from build123d import *

# Parameters (mm, degrees)
SKETCH1_W                 = 100
SKETCH1_H                 = 75
BOSS_EXTRUDE1_DEPTH       = 3.5
F_6_0MM_DOWEL_HOLE5_D     = 6
F_6_0MM_DOWEL_HOLE5_DEPTH = 5.2
F_6_0MM_DOWEL_HOLE5_TIP   = 1.802581857
F_6_0MM_DOWEL_HOLE6_D     = 6
F_6_0MM_DOWEL_HOLE6_DEPTH = 5.2
F_6_0MM_DOWEL_HOLE6_TIP   = 1.802581857
F_6_0MM_DOWEL_HOLE7_D     = 6
F_6_0MM_DOWEL_HOLE7_DEPTH = 5.2
F_6_0MM_DOWEL_HOLE7_TIP   = 1.802581857
F_6_0MM_DOWEL_HOLE8_D     = 6
F_6_0MM_DOWEL_HOLE8_DEPTH = 5.2
F_6_0MM_DOWEL_HOLE8_TIP   = 1.802581857
F_6_0MM_DOWEL_HOLE9_D     = 6
F_6_0MM_DOWEL_HOLE10_D    = 6


with BuildPart() as part:
    # Sketch1 → Boss-Extrude1 (new body)
    with BuildSketch(Plane(origin=(0, 0, 0), x_dir=(1, 0, 0), z_dir=(0, 1, 0))):
        with Locations((-13.448964329, -14.251552142)):
            Rectangle(SKETCH1_W, SKETCH1_H)
    extrude(amount=BOSS_EXTRUDE1_DEPTH)

    # Ø6.0mm Dowel Hole5
    with Locations(Plane(origin=(-137.528418299, 0, 99.034606683), x_dir=(-1, 0, 0), z_dir=(0, -1, 0))):
        with Locations((-154.698850598, 100.900481409)):
            Hole(F_6_0MM_DOWEL_HOLE5_D / 2, depth=F_6_0MM_DOWEL_HOLE5_DEPTH)
            with Locations((0, 0, -(F_6_0MM_DOWEL_HOLE5_DEPTH + F_6_0MM_DOWEL_HOLE5_TIP / 2))):  # 118° drill point
                Cone(0, F_6_0MM_DOWEL_HOLE5_D / 2, F_6_0MM_DOWEL_HOLE5_TIP, mode=Mode.SUBTRACT)

    # Ø6.0mm Dowel Hole6
    with Locations(Plane(origin=(-137.528418299, 0, 99.034606683), x_dir=(-1, 0, 0), z_dir=(0, -1, 0))):
        with Locations((-121.736726509, 100.900481409)):
            Hole(F_6_0MM_DOWEL_HOLE6_D / 2, depth=F_6_0MM_DOWEL_HOLE6_DEPTH)
            with Locations((0, 0, -(F_6_0MM_DOWEL_HOLE6_DEPTH + F_6_0MM_DOWEL_HOLE6_TIP / 2))):  # 118° drill point
                Cone(0, F_6_0MM_DOWEL_HOLE6_D / 2, F_6_0MM_DOWEL_HOLE6_TIP, mode=Mode.SUBTRACT)

    # Ø6.0mm Dowel Hole7
    with Locations(Plane(origin=(-137.528418299, 0, 99.034606683), x_dir=(-1, 0, 0), z_dir=(0, -1, 0))):
        with Locations((-154.698850598, 68.255290468)):
            Hole(F_6_0MM_DOWEL_HOLE7_D / 2, depth=F_6_0MM_DOWEL_HOLE7_DEPTH)
            with Locations((0, 0, -(F_6_0MM_DOWEL_HOLE7_DEPTH + F_6_0MM_DOWEL_HOLE7_TIP / 2))):  # 118° drill point
                Cone(0, F_6_0MM_DOWEL_HOLE7_D / 2, F_6_0MM_DOWEL_HOLE7_TIP, mode=Mode.SUBTRACT)

    # Ø6.0mm Dowel Hole8
    with Locations(Plane(origin=(-137.528418299, 0, 99.034606683), x_dir=(-1, 0, 0), z_dir=(0, -1, 0))):
        with Locations((-121.736726509, 68.255290468)):
            Hole(F_6_0MM_DOWEL_HOLE8_D / 2, depth=F_6_0MM_DOWEL_HOLE8_DEPTH)
            with Locations((0, 0, -(F_6_0MM_DOWEL_HOLE8_DEPTH + F_6_0MM_DOWEL_HOLE8_TIP / 2))):  # 118° drill point
                Cone(0, F_6_0MM_DOWEL_HOLE8_D / 2, F_6_0MM_DOWEL_HOLE8_TIP, mode=Mode.SUBTRACT)

    # Ø6.0mm Dowel Hole9 (through all)
    with Locations(Plane(origin=(-137.528418299, 0, 99.034606683), x_dir=(-1, 0, 0), z_dir=(0, -1, 0))):
        with Locations((-93.346603373, 84.436908191)):
            Hole(F_6_0MM_DOWEL_HOLE9_D / 2)

    # Ø6.0mm Dowel Hole10 (through all)
    with Locations(Plane(origin=(-137.528418299, 0, 99.034606683), x_dir=(-1, 0, 0), z_dir=(0, -1, 0))):
        with Locations((-126.399729662, 84.576636181)):
            Hole(F_6_0MM_DOWEL_HOLE10_D / 2)


solid = part.part
Work out the finished part from the listing and answer in its coordinate system (mm). Give positions to 0.01 mm unless a question says otherwise; leave off trailing zeros. Write each loop counter-clockwise with the first axis right and the second up, starting at its lowest first coordinate (ties: lowest second). Pieces come first, ordered by that corner, then holes. Notation, with made-up numbers: M 57.5,-37 L 91.5,-37 A29 cw 91.5,-17 Z; hole C 56.25,25 d10. An arc over 180 degrees is marked long. Answer as CSV lines item,"result".
Q1. A cutting plane is placed at B-B on z = -3. Write down the section's boundary in (x, y).
A:
outline,"M -63.45,0 L -18.57,0 L -18.57,3.5 L -63.45,3.5 Z; M -13.01,0 L 14.39,0 L 14.39,3.5 L -13.01,3.5 Z; M 19.95,0 L 36.55,0 L 36.55,3.5 L 19.95,3.5 Z"
Q2. The mould has two halves that part along Z. Classify faces 1 (the flat face through (-14, 2, -23.248)), 2 (the flat face through (-14, 3.5, 5)), 3 (the cylindrical face through (-13.34, 1.77, 12.43)): +Z half, -Z half, draft (parallel to the pull), parting line (faces both ways), or undercut.
A:
face 1,"-Z half"
face 2,"draft"
face 3,"undercut"
Q3. A cutting plane is placed at A-A on y = 2.4. Write down the section's boundary in (x, z), plus the area to 3 significant figures.
A:
outline,"M -63.45,-23.25 L 36.55,-23.25 L 36.55,51.75 L -63.45,51.75 Z; hole C -44.18,14.6 d6; hole C -15.79,-1.87 d6; hole C -15.79,30.78 d6; hole C -11.13,14.46 d6; hole C 17.17,-1.87 d6; hole C 17.17,30.78 d6"
area,"7,330 mm²"
Q4. Find the intervals of material crossed by probe 1 along Z at (x, y) = (-14.5, 1.9); probe 2 along X at (y, z) = (2.15, 13); probe 3 along Z at (x, y) = (16.5, 3.4), in increasing order. Write a range as [from, to].
A:
probe 1,"z = [-23.25, -4.57], [0.84, 28.07], [33.49, 51.75]"
probe 2,"x = [-63.45, -46.72], [-41.64, -13.75], [-8.51, 36.55]"
probe 3,"z = [-23.25, -4.79], [1.06, 27.86], [33.7, 51.75]"
